For this review, use the dimensioned drawing (mm, ordinates from the lowest corner) and the shaded views. Coordinates: 2 decimals unless noted, no trailing zeros. Order: outer loops, then holes, each group sorted by start corner. A loop starts at its lowest first (then second) coordinate and runs counter-clockwise, first axis right, second up. Notation, with made-up numbers: (-21.75, 46.25) -> (17.25, 46.25) arc R10 ccw to (17.25, 50.25) -> close; hole circle Ø8 at (-8, 66). An arc over 180 degrees is marked (long way). Return JSON: item names as keys, results as strings. Group by question number.
Item 1: For line 1 along X through (y, z) = (1.85, 10); line 2 along X through (y, z) = (2.95, 11.5); line 3 along Z through (x, y) = (10.5, 2.3), list the stretches that pass through material, from the lowest coordinate up.
Item 2: Take a section at B-B (z = 10). Count the separate pieces of the cut face and the enclosed holes in it, then the cut area to 3 significant figures.
Item 3: Insertion check: pin 1 (1 mm diameter, centred on y = 2, z = 49, fed in from +X); pin 2 (1.5 mm diameter, centred on y = 1.5, z = 32, fed in from +X) (1 decimal); pin 3 (1 mm diameter, centred on y = 1.5, z = 14.5, fed in from -X) (1 decimal). Each pin has a flat end and moves straight along its axis. Give the tip position at first contact, or say it passes through.
Item 4: Take a section at C-C (y = 1). Write out the cut boundary in (x, z), then the cut area to 3 significant figures.
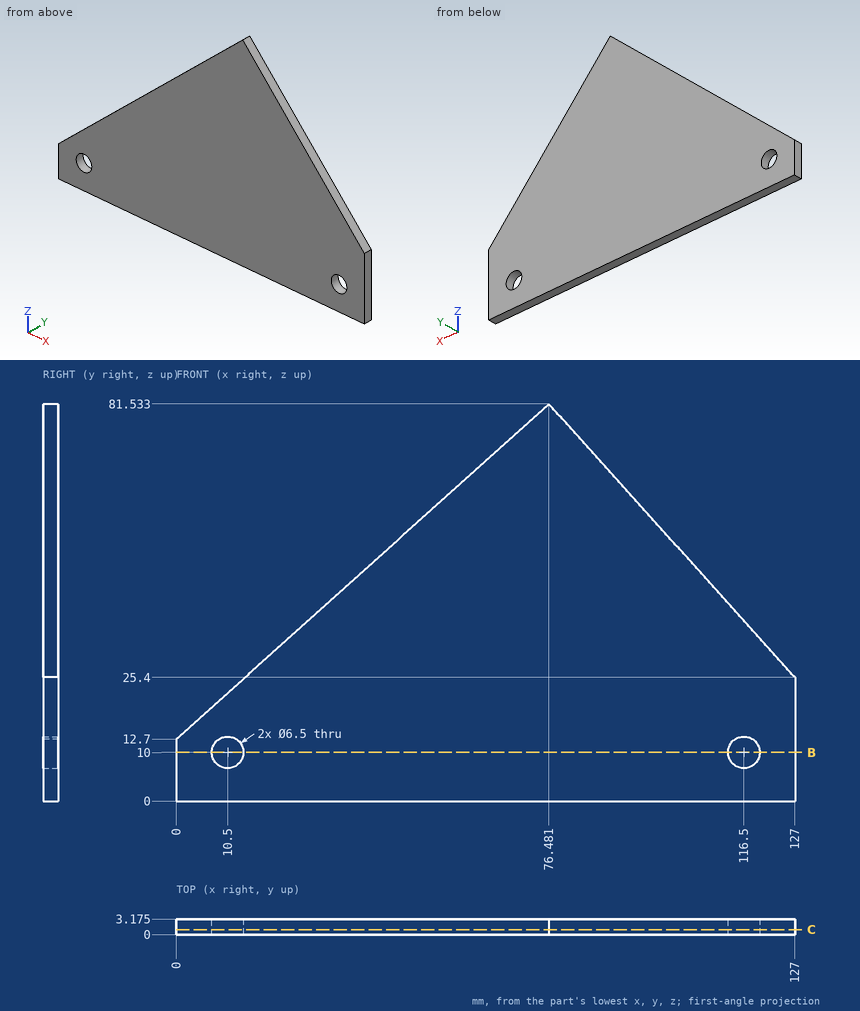
Findings below:
{
 "1": {"line 1": "x = 0 to 7.25, 13.75 to 113.25, 119.75 to 127", "line 2": "x = 0 to 7.62, 13.38 to 113.62, 119.38 to 127", "line 3": "z = 0 to 6.75, 13.25 to 22.15"},
 "2": {"separate pieces": "3", "enclosed holes": "0", "area": "362 mm2"},
 "3": {"pin 1": "stops at x = 106.21", "pin 2": "stops at x = 121.7", "pin 3": "stops at x = 1.4"},
 "4": {"outline": "(0, 0) -> (127, 0) -> (127, 25.4) -> (76.48, 81.53) -> (0, 12.7) -> close; hole circle Ø6.5 at (10.5, 10); hole circle Ø6.5 at (116.5, 10)", "area": "6,240 mm2"}
}
